Autodesk Inventor part; units mm, degrees
ref_plane "YZ Plane" through (0, 0, 0) normal (1, 0, 0) x (0, 1, 0)
ref_plane "XZ Plane" through (0, 0, 0) normal (0, 1, 0) x (-1, 0, 0)
ref_plane "XY Plane" through (0, 0, 0) normal (0, 0, 1) x (1, 0, 0)
sketch "Sketch1" plane through (0, 0, 0) normal (1, 0, 0) x (0, 1, 0)
  circle A0 centre (0, 0) radius 31.75 construction
  circle A1 centre (38.1, 0) radius 6.35
  circle A2 centre (0, 0) radius 18.75 construction
  circle A3 centre (-40.8673, -58.3646) radius 52.5 construction
  circle A4 centre (-40.8673, -58.3646) radius 75 construction
  line L0 (0, 0) -> (0, -31.75) construction
  line L1 (0, 0) -> (38.1, 0) construction
  line L2 (0, 0) -> (-40.8673, -58.3646) construction
  circle A5 centre (38.1, 0) radius 30 construction
  circle A6 centre (-40.8673, -58.3646) radius 14
  circle A7 centre (-13.031, 35.8023) radius 6.35
  line L3 (0, 0) -> (-13.031, 35.8023) construction
  circle A8 centre (-13.031, 35.8023) radius 30 construction
  circle A9 centre (21.8533, 31.2097) radius 6.35
  line L4 (21.8533, 31.2097) -> (0, 0) construction
  circle A10 centre (21.8533, 31.2097) radius 30 construction
  circle A11 centre (-40.8673, 241.6354) radius 75 construction
  line L5 (-40.8673, 241.6354) -> (-40.8673, -58.3646) construction
  circle A12 centre (-40.8673, 241.6354) radius 14
  circle A13 centre (0, 0) radius 9.5
  line L6 (-64.8673, 316.6354) -> (70.1327, 316.6354)
  line L7 (70.1327, 316.6354) -> (70.1327, -133.3646)
  line L8 (70.1327, -133.3646) -> (-64.8673, -133.3646)
  line L9 (-64.8673, -133.3646) -> (-64.8673, 316.6354)
  circle A14 centre (38.1, 0) radius 25.4 construction
  circle A15 centre (38.1, 0) radius 9.7
  circle A16 centre (21.8533, 31.2097) radius 9.7
  circle A17 centre (-13.031, 35.8023) radius 9.7
  dimension "d0" = 63.5
  dimension "d1" = 12.7
  dimension "d2" = 37.5
  dimension "d3" = 105
  dimension "d4" = 150
  dimension "d5" = 90
  dimension "d6" = 35
  dimension "d7" = 60
  dimension "d8" = 28
  dimension "d9" = 12.7
  dimension "d10" = 60
  dimension "d11" = 200
  dimension "d13" = 12.7
  dimension "d14" = 145
  dimension "d15" = 60
  dimension "d16" = 150
  dimension "d17" = 300
  dimension "d18" = 28
  dimension "d19" = 19
  dimension "d20" = 135
  dimension "d21" = 450
  dimension "d22" = 24
  dimension "d23" = 75
  dimension "d24" = 50.8
  dimension "d25" = 19.4
  dimension "d26" = 19.4
  dimension "d27" = 19.4
extrude "Extrusion1" add sketch "Sketch1" along normal blind 7 contours L6 L7 L8 L9
sketch "Cheese" plane through (7, 0, 0) normal (1, 0, 0) x (0, 0, -1)
  line L0 (-316.6354, 70.1327) -> (-81.6354, 70.1327)
  line L1 (-81.6354, 70.1327) -> (-81.6354, -0.8673)
  line L2 (-81.6354, -0.8673) -> (-316.6354, -0.8673)
  line L3 (-316.6354, -0.8673) -> (-316.6354, 70.1327)
  circle A0 centre (-241.6354, -40.8673) radius 14
  line L4 (-81.6354, 70.1327) -> (-141.2115, -0.8673)
  line L5 (133.3646, 70.1327) -> (-316.6354, 70.1327)
  line L6 (133.3646, 70.1327) -> (43.3646, 70.1327)
  line L7 (43.3646, 70.1327) -> (43.3646, -0.8673)
  line L8 (43.3646, -0.8673) -> (133.3646, -0.8673)
  line L9 (133.3646, -0.8673) -> (133.3646, 70.1327)
  circle A1 centre (58.3646, -40.8673) radius 14
  line L10 (43.3646, 70.1327) -> (102.9407, -0.8673)
  circle A2 centre (-241.6354, -40.8673) radius 24
  circle A3 centre (58.3646, -40.8673) radius 24
  line L11 (-296.7727, -10.8673) -> (-252.6928, -10.8673) construction
  line L12 (-81.6354, 70.1327) -> (-141.2115, -0.8673)
  line L13 (-316.6354, 70.1327) -> (-316.6354, -64.8673)
  line L14 (-316.6354, -0.8673) -> (-316.6354, 70.1327)
  line L15 (-316.6354, 70.1327) -> (-81.6354, 70.1327)
  line L16 (102.9407, -0.8673) -> (43.3646, 70.1327)
  line L17 (133.3646, 70.1327) -> (43.3646, 70.1327)
  line L18 (133.3646, 70.1327) -> (133.3646, -0.8673)
  line L19 (102.9407, -0.8673) -> (133.3646, -0.8673)
  line L20 (-141.2115, -0.8673) -> (-81.6354, 70.1327)
  line L21 (-316.6354, 70.1327) -> (-81.6354, 70.1327)
  line L22 (-316.6354, 70.1327) -> (-316.6354, -0.8673)
  line L23 (-316.6354, -0.8673) -> (-141.2115, -0.8673)
  line L24 (43.3646, 70.1327) -> (133.3646, 70.1327)
  line L25 (133.3646, -0.8673) -> (133.3646, 70.1327)
  line L26 (43.3646, 70.1327) -> (102.9407, -0.8673)
  line L27 (102.9407, -0.8673) -> (133.3646, -0.8673)
  line L28 (133.3646, -64.8673) -> (133.3646, 70.1327)
  point P0 (0, 0)
  dimension "d30" = 40
  dimension "d32" = 40
  dimension "d33" = 71
  dimension "d34" = 71
  dimension "d35" = 40
  dimension "d36" = 90
  dimension "d37" = 40
  dimension "d38" = 48
  dimension "d39" = 48
  dimension "d44" = 125
extrude "Extrusion2" cut sketch "Cheese" against normal blind 7 contours L5 L9 L8 L10 | L0 L4 L2 L3
sketch "Sketch3" plane through (7, 0, 0) normal (1, 0, 0) x (0, 0, -1)
  circle A0 centre (-106.8994, 15.1327) radius 3.25
  circle A1 centre (35.9037, 54.1327) radius 3.25
  circle A2 centre (68.6285, 15.1327) radius 3.25
  circle A3 centre (-296.3854, -16.8673) radius 3.25
  circle A4 centre (-296.3854, -48.8673) radius 3.25
  circle A5 centre (-74.1745, 54.1327) radius 3.25
  line L0 (-316.6354, -0.8673) -> (-316.6354, -64.8673)
  line L1 (-316.6354, -64.8673) -> (133.3646, -64.8673)
  line L2 (-141.2115, -0.8673) -> (-316.6354, -0.8673)
  circle A6 centre (-237.8854, -16.8673) radius 3.25
  circle A7 centre (-237.8854, -48.8673) radius 3.25
  circle A8 centre (-179.3854, -16.8673) radius 3.25
  circle A9 centre (-179.3854, -48.8673) radius 3.25
  circle A10 centre (-120.8854, -16.8673) radius 3.25
  circle A11 centre (-120.8854, -48.8673) radius 3.25
  circle A12 centre (-62.3854, -16.8673) radius 3.25
  circle A13 centre (-62.3854, -48.8673) radius 3.25
  circle A14 centre (-3.8854, -16.8673) radius 3.25
  circle A15 centre (-3.8854, -48.8673) radius 3.25
  circle A16 centre (54.6146, -16.8673) radius 3.25
  circle A17 centre (54.6146, -48.8673) radius 3.25
  circle A18 centre (113.1146, -16.8673) radius 3.25
  circle A19 centre (113.1146, -48.8673) radius 3.25
  line L3 (43.3646, 70.1327) -> (-81.6354, 70.1327)
  line L4 (-81.6354, 70.1327) -> (-141.2115, -0.8673)
  line L5 (102.9407, -0.8673) -> (43.3646, 70.1327)
  line L6 (133.3646, -0.8673) -> (102.9407, -0.8673)
  circle A20 centre (125.3646, -56.8673) radius 3.25
  line L7 (133.3646, -64.8673) -> (133.3646, -0.8673)
  circle A21 centre (125.3646, -8.8673) radius 3.25
  circle A22 centre (-31.2097, 21.8533) radius 25.4 construction
  circle A23 centre (-31.2097, 21.8533) radius 9.7
  circle A24 centre (0, 38.1) radius 25.4 construction
  circle A25 centre (0, 38.1) radius 9.7
  circle A26 centre (-35.8023, -13.031) radius 25.4 construction
  circle A27 centre (-35.8023, -13.031) radius 9.7
  circle A28 centre (12.3646, 60.2873) radius 2.75
  circle A29 centre (-13.0325, 59.9017) radius 2.75
  circle A30 centre (-25.3971, 37.7144) radius 2.75
  circle A31 centre (-12.3646, 15.9127) radius 2.75
  circle A32 centre (13.0325, 16.2983) radius 2.75
  circle A33 centre (25.3971, 38.4856) radius 2.75
  circle A34 centre (-42.6354, 44.5383) radius 2.75
  circle A35 centre (-56.5684, 23.3008) radius 2.75
  circle A36 centre (-45.1427, 0.6158) radius 2.75
  circle A37 centre (-19.784, -0.8318) radius 2.75
  circle A38 centre (-5.851, 20.4057) radius 2.75
  circle A39 centre (-17.2767, 43.0908) radius 2.75
  circle A40 centre (-25.7736, -36.3673) radius 2.75
  circle A41 centre (-10.5781, -16.014) radius 2.75
  circle A42 centre (-20.6068, 7.3223) radius 2.75
  circle A43 centre (-45.831, 10.3054) radius 2.75
  circle A44 centre (-61.0265, -10.0479) radius 2.75
  circle A45 centre (-50.9978, -33.3842) radius 2.75
  point P0 (0, 0)
  dimension "d33" = 71
  dimension "d34" = 71
  dimension "d182" = 50.8
  dimension "d183" = 50.8
  dimension "d184" = 50.8
  dimension "d47" = 6.5
  dimension "d48" = 6.5
  dimension "d49" = 6.5
  dimension "d52" = 6.5
  dimension "d53" = 6.5
  dimension "d54" = 6.5
  dimension "d55" = 20.25
  dimension "d56" = 20.25
  dimension "d57" = 16
  dimension "d58" = 16
  dimension "d61" = 58.5
  dimension "d66" = 16
  dimension "d67" = 16
  dimension "d68" = 16
  dimension "d69" = 16
  dimension "d70" = 16
  dimension "d71" = 16
  dimension "d72" = 16
  dimension "d73" = 16
  dimension "d91" = 6.5
  dimension "d92" = 8
  dimension "d93" = 8
  dimension "d179" = 6.5
  dimension "d180" = 8
  dimension "d181" = 8
  dimension "d185" = 5.5
  dimension "d188" = 360
  dimension "d190" = 31
  dimension "d191" = 5.5
  dimension "d194" = 360
  dimension "d196" = 39
  dimension "d197" = 5.5
  dimension "d200" = 360
  dimension "d202" = 28.5
extrude "Extrusion3" cut sketch "Sketch3" against normal blind 7 contours A0 | A1 | A3 | A4 | A5 | A8 | A9 | A13 | A20 | A21 | A28 | A29 | A30 | A31 | A32 | A33 | A34 | A35 | A36 | A37 | A38 | A39 | A40 | A41 | A42 | A43 | A44 | A45
sketch "Sketch6" plane through (7, 0, 0) normal (1, 0, 0) x (0, 0, -1)
  circle A0 centre (-81.6354, 10.1327) radius 15
  line L0 (43.3646, 70.1327) -> (-81.6354, 70.1327)
  line L1 (133.3646, -64.8673) -> (133.3646, -0.8673)
  line L2 (-81.6354, 70.1327) -> (-141.2115, -0.8673)
  circle A1 centre (48.3646, 9.1327) radius 30
  line L3 (-316.6354, -64.8673) -> (133.3646, -64.8673)
  circle A2 centre (103.3646, -29.8673) radius 20
  circle A3 centre (13.3646, -37.8673) radius 17.5
  circle A4 centre (-136.6354, -32.8673) radius 24
  line L4 (-316.6354, -0.8673) -> (-316.6354, -64.8673)
  circle A5 centre (-86.6354, -35.8673) radius 15
  line L5 (-141.2115, -0.8673) -> (-316.6354, -0.8673)
  circle A6 centre (-201.6354, -32.8673) radius 17
  circle A7 centre (-276.6354, -32.8673) radius 15
  circle A8 centre (-249.6354, -12.8673) radius 8.5
  circle A9 centre (-227.6354, -16.8673) radius 8.5
  circle A10 centre (-89.0925, 44.1327) radius 5
  circle A11 centre (-264.6354, -54.8673) radius 5.5
  circle A12 centre (-106.6354, -9.8673) radius 7
  circle A13 centre (-36.6354, 60.1327) radius 7.5
  circle A14 centre (-62.6354, 40.1327) radius 8.5
  circle A15 centre (-36.6354, -49.8673) radius 9
  point P0 (0, 0)
  dimension "d123" = 30
  dimension "d124" = 60
  dimension "d125" = 215
  dimension "d129" = 60
  dimension "d130" = 85
  dimension "d131" = 74
  dimension "d132" = 40
  dimension "d133" = 30
  dimension "d134" = 35
  dimension "d136" = 35
  dimension "d137" = 120
  dimension "d138" = 27
  dimension "d144" = 48
  dimension "d145" = 32
  dimension "d146" = 180
  dimension "d147" = 30
  dimension "d148" = 230
  dimension "d149" = 35
  dimension "d156" = 34
  dimension "d157" = 32
  dimension "d158" = 115
  dimension "d159" = 30
  dimension "d160" = 40
  dimension "d161" = 32
  dimension "d162" = 17
  dimension "d163" = 17
  dimension "d164" = 67
  dimension "d165" = 12
  dimension "d166" = 89
  dimension "d167" = 16
  dimension "d168" = 10
  dimension "d169" = 11
  dimension "d170" = 26
  dimension "d171" = 11
  dimension "d172" = 52
  dimension "d173" = 10
  dimension "d176" = 14
  dimension "d177" = 210
  dimension "d178" = 55
  dimension "d203" = 15
  dimension "d204" = 10
  dimension "d205" = 45
  dimension "d206" = 17
  dimension "d207" = 19
  dimension "d208" = 30
  dimension "d209" = 18
  dimension "d210" = 170
  dimension "d211" = 15
extrude "Extrusion4" cut sketch "Sketch6" against normal blind 10
fillet "Fillet2" radius 10 4 edges at (3.5, -0.8673, 141.2115) (3.5, 70.1327, 81.6354) (3.5, 70.1327, -43.3646) (3.5, -0.8673, -102.9407)
sketch "Sketch7" plane through (0, -0.8673, 316.6354) normal (0, 1, 0) x (1, 0, 0)
  circle A0 centre (3.5, 10) radius 2.1
  line L0 (0, 0) -> (0, 170.7608)
  line L1 (7, 0) -> (0, 0)
  circle A1 centre (3.5, 40) radius 2.1
  circle A2 centre (4.2231, 150) radius 2.1
  point P0 (0, 316.6354)
  dimension "d213" = 4.2
  dimension "d214" = 3.5
  dimension "d215" = 10
  dimension "d221" = 4.2
  dimension "d222" = 3.5
  dimension "d223" = 40
  dimension "d224" = 4.2
  dimension "d225" = 150
extrude "Extrusion5" cut sketch "Sketch7" against normal blind 10
sketch "Sketch8" plane through (0, -64.8673, 316.6354) normal (0, 0, 1) x (1, 0, 0)
  line L0 (0, 0) -> (7, 0)
  line L1 (7, 64) -> (0, 64)
  line L2 (7, 0) -> (0, 0)
  line L3 (0, 0) -> (0, 64)
  line L4 (0, 64) -> (7, 64)
  line L5 (7, 64) -> (7, 0)
  point P0 (0, 64.8673)
  dimension "d226" = 7
  dimension "d227" = 64
extrude "Front" add sketch "Sketch8" along normal blind 200
sketch "Sketch9" plane through (7, -64.8673, -133.3646) normal (0, 0, -1) x (-1, 0, 0)
  line L0 (0, 64) -> (7, 64)
  line L1 (7, 64) -> (0, 64)
  line L2 (0, 64) -> (0, 0)
  line L3 (0, 0) -> (7, 0)
  line L4 (7, 0) -> (7, 64)
  point P0 (7, 64.8673)
  dimension "d230" = 64
  dimension "d231" = 7
extrude "Extrusion7" add sketch "Sketch9" along normal blind 200
equation "\"d9\" = d1"
equation "\"d13\" = d1"
equation "\"d14\" = 0.5 * d5 + 0.5 * d11"
equation "\"d16\" = d4"
equation "\"d18\" = d8"
equation "\"d26\" = d25"
equation "\"d27\" = d25"
equation "\"d34\" = d33"
equation "\"d35\" = d30"
equation "\"d56\" = d55"
equation "\"d58\" = d57"
properties part number "Cheese" material "Aluminum 6061"
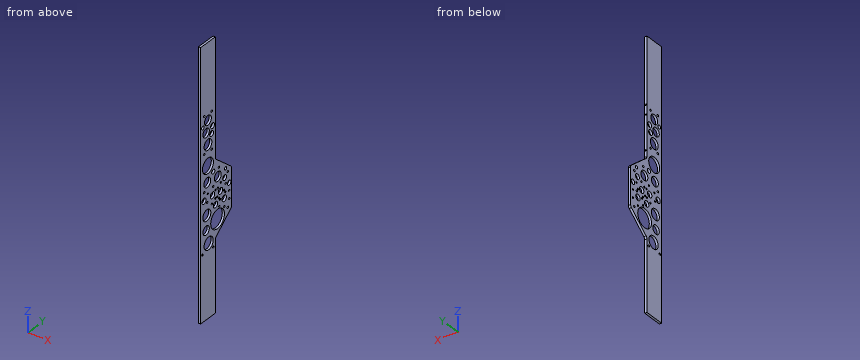
Build history of the part. All positions in model axes, mm. Round coordinates to 2 decimals unless told otherwise and drop trailing zeros. Order: outer loops, then holes, each group sorted by start corner. A loop starts at its lowest first (then second) coordinate and runs counter-clockwise, first axis right, second up. Notation, with made-up numbers: (71, 36.5) -> (83, 36.5) arc R20 ccw to (83, 74.5) -> close; hole circle Ø7 at (41.5, 20). An arc over 180 degrees is marked (long way). Answer in a Markdown table with one row per item.
1) Band-saw the part on A-A on z = -257.5. Give the cut face in (x, y).
Values:
| item | result |
|---|---|
| outline | (0, -64.87) -> (7, -64.87) -> (7, -0.87) -> (0, -0.87) -> close |
2) Band-saw the part on B-B on x = 4. Give the number of separate pieces and of enclosed holes in the cut face, and give its area (3 significant figures).
Values:
| item | result |
|---|---|
| separate pieces | 1 |
| enclosed holes | 50 |
| area | 52,900 mm2 |
3) Pin check, flat tips, straight feed: P1, Ø9, axis at y = -54.87, z = 264.64, coming from the +X side; P2, Ø3.5, axis at x = 3.5, z = 307.5, coming from the +Y side; P3, Ø1, axis at x = 1, y = 22.5, coming from the -Z side. Stop position of each tip, or through.
Values:
| item | result |
|---|---|
| P1 | through |
| P2 | y = -0.87 |
| P3 | z = -83.75 |
4) Wall check: L1, parallel to Y at x = 5.25, z = 241; L2, parallel to Z at x = 3.5, y = 24; L3, parallel to Z at x = 2, y = 13.5 (3 decimals). Give the ranges that are in metal, low to high.
Values:
| item | result |
|---|---|
| L1 | -64.87 to -54.85, -26.88 to -0.87 |
| L2 | -82.07 to -74.42, -22.31 to 21.75, 40.67 to 53.91, 59.23 to 75.92, 87.35 to 120.35 |
| L3 | -90.885 to -78.045, -18.684 to 11.045, 13.684 to 26.279, 36.14 to 67.018, 96.253 to 104.089, 109.71 to 129.156 |
